For this review, take the finished solid that the model builds, in its own axes (mm). Round coordinates to 2 decimals unless told otherwise and drop trailing zeros. Order: outer loops, then holes, each group sorted by start corner. A loop starts at its lowest first (then second) coordinate and runs counter-clockwise, first axis right, second up.
from build123d import *

# Parameters (mm, degrees)
SKETCH1_R           = 108.978645108
SKETCH1_R_2         = 82.075459911
BOSS_EXTRUDE1_DEPTH = 5
SKETCH3_W           = 27.601566605
SKETCH3_H           = 5
CUT_EXTRUDE1_DEPTH  = 5
CIRPATTERN1_COUNT   = 12


with BuildPart() as part:
    # Sketch1 → Boss-Extrude1 (new body)
    with BuildSketch(Plane(origin=(0, 0, 0), x_dir=(1, 0, 0), z_dir=(0, 1, 0))):
        Circle(SKETCH1_R)
        Circle(SKETCH1_R_2, mode=Mode.SUBTRACT)
    extrude(amount=BOSS_EXTRUDE1_DEPTH)

    # Sketch2 → Cut-Revolve1 (revolve, cut)
    with BuildSketch(Plane.XY):
        Polygon((108.978645108, 0), (108.468178891, 15.211545536), (125.564128825, 15.211545536), (125.564128825, 0), align=None)
    revolve(axis=Axis((0, 0, 0), (0, 1, 0)), mode=Mode.SUBTRACT)

    # Sketch3 → Cut-Extrude1 (cut)
    with BuildSketch(Plane(origin=(0, 5, 0), x_dir=(1, 0, 0), z_dir=(0, 1, 0))):
        with Locations((85.467576893, 0)):
            Rectangle(SKETCH3_W, SKETCH3_H)
    cut_extrude1 = extrude(amount=-CUT_EXTRUDE1_DEPTH, mode=Mode.SUBTRACT)

    # CirPattern1: Cut-Extrude1 ×12 about axis
    cirpattern1_axis = Axis((0, 0, 0), (0, 1, 0))
    for i in range(1, CIRPATTERN1_COUNT):
        add(cut_extrude1.rotate(cirpattern1_axis, i * 360 / CIRPATTERN1_COUNT), mode=Mode.SUBTRACT)


solid = part.part
(1) Wall thickness on L1, parallel to Z at x = 75, y = 4.5; L2, parallel to X at y = 2.45, z = -76; L3, parallel to Z at x = -15.5, y = 3.15: over which ranges is each line inside the solid? List them lowest first.
(2) Add section B-B on x = 0. Give the boundary of the cut face in (y, z).
(3) Draft analysis for pull direction Z (two halves, no side actions). For faces 1 (the face through (-17, 0, -81)), 2 (the face through (-91, 3, 2.5)), state which applies: pulls with the +Z half, pulls with the -Z half, needs draft (parallel to the pull), parting line crosses it, or undercut.
(4) Clearance check with flat-ended pins moving along their axes: P1, Ø2.5, axis at x = -0.5, y = 3.5, coming from the -Z side; P2, Ø4, axis at x = 67, z = 76, coming from the -Y side; P3, Ø2.5, axis at x = 95, y = 1.5, coming from the +Z side; P4, Ø2.5, axis at y = 1.5, z = -93, coming from the +X side. State where each tip first meets the part, or that it passes through.
(5) Add section A-A on z = 0. Give the boundary of the cut face in (x, y).
Here are the results:
1. L1: z = -78.86 to -46.19, -40.41 to -33.34, 33.34 to 40.41, 46.19 to 78.86
1. L2: x = -77.99 to -46.77, -40.99 to -30.99, 30.99 to 40.99, 46.77 to 77.99
1. L3: z = -107.76 to -80.6, 80.6 to 107.76
2. outline: (0, -108.98) - (5, -108.81) - (5, -99.27) - (0, -99.27) - close; (0, 99.27) - (5, 99.27) - (5, 108.81) - (0, 108.98) - close
3. face 1: needs draft
3. face 2: undercut
4. P1: stops at z = -108.9
4. P2: stops at y = 0
4. P3: stops at z = 55.47
4. P4: stops at x = 58.72
5. outline: (-108.98, 0) - (-99.27, 0) - (-99.27, 5) - (-108.81, 5) - close; (99.27, 0) - (108.98, 0) - (108.81, 5) - (99.27, 5) - close
